Verification items for the finished model (mm, model axes). Face numbers are marked on the shaded views. A direction names the side the tool comes from. Coordinates: 2 decimals unless noted, no trailing zeros. Order: outer loops, then holes, each group sorted by start corner. A loop starts at its lowest first (then second) coordinate and runs counter-clockwise, first axis right, second up.
Q1. Thickness scan on line 1 (X direction, y = 13, z = 11.5); line 2 (X direction, y = 12, z = 27.5); line 3 (Z direction, x = 9, y = -3.5). Record the ranges inside material, lowest first.
Q2. Draft check along Y on the marked faces 1, 2, 3 and 4. Enter one of: pulls with the +Y half, pulls with the -Y half, needs draft (parallel to the pull), parting line crosses it, or undercut.
Q3. Cross-section at C-C, the plane y = -9. Record the boundary of the cut face in (x, z), and give its area (3 significant figures).
Q4. Cross-section at A-A, the plane z = 35. Record the boundary of the cut face in (x, y).
Q5. Depth check by flat-ended pin: P1, Ø2, axis at x = 12, z = 39, coming from the -Y side; P2, Ø2, axis at x = 6.5, z = 49, coming from the -Y side; P3, Ø2, axis at x = -5, y = -10.5, coming from the -Z side. Enter the tip coordinate at first touch or a pass-through.
Q6. Cross-section at D-D, the plane y = -13.5. Record the boundary of the cut face in (x, z), and give its area (3 significant figures).
Q7. Set-up check for the marked faces 5, 6, 7, 8 and 9: record each of +Z, -Z, +X, -X, +Y, -Y from which the full face is reachable in a straight line by a thin tool's end or side.
Q8. Cross-section at B-B, the plane x = -4. Record the boundary of the cut face in (y, z), and give its area (3 significant figures).
from build123d import *

# Parameters (mm, degrees)
F1_DEPTH = 60
F2_T     = -1
F4_DEPTH = 59
F6_DEPTH = 2


with BuildPart() as f1:
    # F0 (on Top) → F1 (new body)
    with BuildSketch(Plane.XY):
        Polygon((-7.2654252801, 15), (-14.5308505601, 20), (-12.0207078615, 11.5450849719), (-10.8981379201, 15), align=None)
        Polygon((-10.8981379201, 15), (-12.0207078615, 11.5450849719), (-9.510565163, 3.0901699437), (-16.5109876273, -2.2745751406), (-17.6335575688, -5.7294901688), (-14.6946313073, -7.8647450844), (-5.8778525229, -8.0901699437), (-2.9389262615, -16.4057647469), (0, -18.5410196625), (2.9389262615, -16.4057647469), (5.8778525229, -8.0901699437), (14.6946313073, -7.8647450844), (17.6335575688, -5.7294901688), (16.5109876273, -2.2745751406), (9.510565163, 3.0901699437), (12.0207078615, 11.5450849719), (10.8981379201, 15), (7.2654252801, 15), (0, 10), (-7.2654252801, 15), align=None)
        Polygon((-9.510565163, 3.0901699437), (-12.0207078615, 11.5450849719), (-16.5109876273, -2.2745751406), align=None)
        Polygon((7.2654252801, 15), (-7.2654252801, 15), (0, 10), align=None)
        Polygon((-17.6335575688, -5.7294901688), (-16.5109876273, -2.2745751406), (-23.5114100917, -7.639320225), (-14.6946313073, -7.8647450844), align=None)
        Polygon((14.5308505601, 20), (7.2654252801, 15), (10.8981379201, 15), (12.0207078615, 11.5450849719), align=None)
        Polygon((-5.8778525229, -8.0901699437), (-14.6946313073, -7.8647450844), (-2.9389262615, -16.4057647469), align=None)
        Polygon((16.5109876273, -2.2745751406), (12.0207078615, 11.5450849719), (9.510565163, 3.0901699437), align=None)
        Polygon((0, -18.5410196625), (-2.9389262615, -16.4057647469), (0, -24.72135955), (2.9389262615, -16.4057647469), align=None)
        Polygon((23.5114100917, -7.639320225), (16.5109876273, -2.2745751406), (17.6335575688, -5.7294901688), (14.6946313073, -7.8647450844), align=None)
        Polygon((5.8778525229, -8.0901699437), (2.9389262615, -16.4057647469), (14.6946313073, -7.8647450844), align=None)
    extrude(amount=F1_DEPTH)

    # F2
    f2_openings = [f1.faces().sort_by_distance(p)[0] for p in [
        (0, 0, 0),
    ]]
    offset(amount=F2_T, openings=f2_openings, kind=Kind.INTERSECTION)

    # F3 (on face) → F4 (join, through all)
    with BuildSketch(Plane(origin=(0, 0, 59), x_dir=(1, 0, 0), z_dir=(0, 0, -1))):
        Polygon((-15.6559881063, 2.8792251681), (-14.3583265336, 6.8730168274), (-20.6573081254, 6.7119662811), align=None)
        Polygon((0, 21.7203791484), (-2.0996605306, 15.7794590151), (2.0996605306, 15.7794590151), align=None)
        Polygon((20.6573081254, 6.7119662811), (14.3583265336, 6.8730168274), (15.6559881063, 2.8792251681), align=None)
        Polygon((12.7669185376, -17.5721558553), (10.9735943499, -11.5317010106), (7.5762722465, -14), align=None)
        Polygon((-7.5762722465, -14), (-10.9735943499, -11.5317010106), (-12.7669185376, -17.5721558553), align=None)
    extrude(amount=F4_DEPTH)

    # F5 (on face) → F6 (join)
    with BuildSketch(Plane(origin=(0, 0, 59), x_dir=(1, 0, 0), z_dir=(0, 0, -1))):
        with BuildLine():
            ThreePointArc((-1.9818535798, 1.8771366278), (-2.208391982, 1.6044906934), (-2.3976894584, 1.3047876426))
            Line((-2.3976894584, 1.3047876426), (-1.3090169944, 0.9510565163))
            Line((-1.3090169944, 0.9510565163), (-1.9818535798, 1.8771366278))
        make_face()
        with BuildLine():
            Line((-1.3090169944, 0.9510565163), (-2.3976894584, 1.3047876426))
            ThreePointArc((-2.3976894584, 1.3047876426), (-2.5961204766, 0.8435306766), (-2.7067064528, 0.3537311263))
            Line((-2.7067064528, 0.3537311263), (-1.6180339887, 0))
            Line((-1.6180339887, 0), (-2.7067064528, -0.3537311263))
            ThreePointArc((-2.7067064528, -0.3537311263), (-2.5961204766, -0.8435306766), (-2.3976894584, -1.3047876426))
            Line((-2.3976894584, -1.3047876426), (-1.3090169944, -0.9510565163))
            Line((-1.3090169944, -0.9510565163), (-1.9818535798, -1.8771366278))
            ThreePointArc((-1.9818535798, -1.8771366278), (-1.6044906934, -2.208391982), (-1.1728365854, -2.4649218801))
            Line((-1.1728365854, -2.4649218801), (-0.5, -1.5388417686))
            Line((-0.5, -1.5388417686), (-0.5, -2.6835397391))
            ThreePointArc((-0.5, -2.6835397391), (1.21e-08, -2.7297226107), (0.5000000237, -2.6835397347))
            Line((0.5000000237, -2.6835397347), (0.5000000237, -1.5388418013))
            Line((0.5000000237, -1.5388418013), (1.1728365854, -2.4649218801))
            ThreePointArc((1.1728365854, -2.4649218801), (1.6044906934, -2.208391982), (1.9818535798, -1.8771366278))
            Line((1.9818535798, -1.8771366278), (1.3090169944, -0.9510565163))
            Line((1.3090169944, -0.9510565163), (2.3976894584, -1.3047876426))
            ThreePointArc((2.3976894584, -1.3047876426), (2.5961204766, -0.8435306766), (2.7067064528, -0.3537311263))
            Line((2.7067064528, -0.3537311263), (1.6180339887, 0))
            Line((1.6180339887, 0), (2.7067064528, 0.3537311263))
            ThreePointArc((2.7067064528, 0.3537311263), (2.5961204766, 0.8435306766), (2.3976894584, 1.3047876426))
            Line((2.3976894584, 1.3047876426), (1.3090169944, 0.9510565163))
            Line((1.3090169944, 0.9510565163), (1.9818535798, 1.8771366278))
            ThreePointArc((1.9818535798, 1.8771366278), (1.6044906934, 2.208391982), (1.1728365854, 2.4649218801))
            Line((1.1728365854, 2.4649218801), (0.5, 1.5388417686))
            Line((0.5, 1.5388417686), (0.5, 2.6835397391))
            ThreePointArc((0.5, 2.6835397391), (0, 2.7297226107), (-0.5, 2.6835397391))
            Line((-0.5, 2.6835397391), (-0.5, 1.5388417686))
            Line((-0.5, 1.5388417686), (-1.1728365854, 2.4649218801))
            ThreePointArc((-1.1728365854, 2.4649218801), (-1.6044906934, 2.208391982), (-1.9818535798, 1.8771366278))
            Line((-1.9818535798, 1.8771366278), (-1.3090169944, 0.9510565163))
        make_face()
        with BuildLine():
            Line((-1.6180339887, 0), (-2.7067064528, 0.3537311263))
            ThreePointArc((-2.7067064528, 0.3537311263), (-2.7297226107, 0), (-2.7067064528, -0.3537311263))
            Line((-2.7067064528, -0.3537311263), (-1.6180339887, 0))
        make_face()
        with BuildLine():
            ThreePointArc((-0.5, 2.6835397391), (-0.8435306766, 2.5961204766), (-1.1728365854, 2.4649218801))
            Line((-1.1728365854, 2.4649218801), (-0.5, 1.5388417686))
            Line((-0.5, 1.5388417686), (-0.5, 2.6835397391))
        make_face()
        with BuildLine():
            Line((-1.3090169944, -0.9510565163), (-2.3976894584, -1.3047876426))
            ThreePointArc((-2.3976894584, -1.3047876426), (-2.208391982, -1.6044906934), (-1.9818535798, -1.8771366278))
            Line((-1.9818535798, -1.8771366278), (-1.3090169944, -0.9510565163))
        make_face()
        with BuildLine():
            ThreePointArc((1.1728365854, 2.4649218801), (0.8435306766, 2.5961204766), (0.5, 2.6835397391))
            Line((0.5, 2.6835397391), (0.5, 1.5388417686))
            Line((0.5, 1.5388417686), (1.1728365854, 2.4649218801))
        make_face()
        with BuildLine():
            Line((-0.5, -1.5388417686), (-1.1728365854, -2.4649218801))
            ThreePointArc((-1.1728365854, -2.4649218801), (-0.8435306766, -2.5961204766), (-0.5, -2.6835397391))
            Line((-0.5, -2.6835397391), (-0.5, -1.5388417686))
        make_face()
        with BuildLine():
            ThreePointArc((2.3976894584, 1.3047876426), (2.208391982, 1.6044906934), (1.9818535798, 1.8771366278))
            Line((1.9818535798, 1.8771366278), (1.3090169944, 0.9510565163))
            Line((1.3090169944, 0.9510565163), (2.3976894584, 1.3047876426))
        make_face()
        with BuildLine():
            Line((0.5000000237, -1.5388418013), (0.5000000237, -2.6835397347))
            ThreePointArc((0.5000000237, -2.6835397347), (0.8435306881, -2.5961204728), (1.1728365854, -2.4649218801))
            Line((1.1728365854, -2.4649218801), (0.5000000237, -1.5388418013))
        make_face()
        with BuildLine():
            ThreePointArc((2.7297226107, 0), (2.7239624938, 0.1772395647), (2.7067064528, 0.3537311263))
            Line((2.7067064528, 0.3537311263), (1.6180339887, 0))
            Line((1.6180339887, 0), (2.7067064528, -0.3537311263))
            ThreePointArc((2.7067064528, -0.3537311263), (2.7239624938, -0.1772395647), (2.7297226107, 0))
        make_face()
        with BuildLine():
            Line((1.3090169944, -0.9510565163), (1.9818535798, -1.8771366278))
            ThreePointArc((1.9818535798, -1.8771366278), (2.208391982, -1.6044906934), (2.3976894584, -1.3047876426))
            Line((2.3976894584, -1.3047876426), (1.3090169944, -0.9510565163))
        make_face()
        with BuildLine():
            Line((-2.3976894584, 1.3047876426), (-14.8526488228, 5.3516492559))
            Line((-14.8526488228, 5.3516492559), (-15.1616658171, 4.4005927396))
            Line((-15.1616658171, 4.4005927396), (-2.7067064528, 0.3537311263))
            ThreePointArc((-2.7067064528, 0.3537311263), (-2.5961204766, 0.8435306766), (-2.3976894584, 1.3047876426))
        make_face()
        with BuildLine():
            Line((-8.6335020293, 11.0323452951), (-1.9818535798, 1.8771366278))
            ThreePointArc((-1.9818535798, 1.8771366278), (-1.6044906934, 2.208391982), (-1.1728365854, 2.4649218801))
            Line((-1.1728365854, 2.4649218801), (-7.8244850349, 11.6201305474))
            Line((-7.8244850349, 11.6201305474), (-8.6335020293, 11.0323452951))
        make_face()
        with BuildLine():
            Line((-0.5, 15.7794590151), (-0.5, 2.6835397391))
            ThreePointArc((-0.5, 2.6835397391), (0, 2.7297226107), (0.5, 2.6835397391))
            Line((0.5, 2.6835397391), (0.5, 15.7794590151))
            Line((0.5, 15.7794590151), (-0.5, 15.7794590151))
        make_face()
        with BuildLine():
            Line((7.8244850349, 11.6201305474), (1.1728365854, 2.4649218801))
            ThreePointArc((1.1728365854, 2.4649218801), (1.6044906934, 2.208391982), (1.9818535798, 1.8771366278))
            Line((1.9818535798, 1.8771366278), (8.6335020293, 11.0323452951))
            Line((8.6335020293, 11.0323452951), (7.8244850349, 11.6201305474))
        make_face()
        with BuildLine():
            Line((14.8526488228, 5.3516492559), (2.3976894584, 1.3047876426))
            ThreePointArc((2.3976894584, 1.3047876426), (2.5961204766, 0.8435306766), (2.7067064528, 0.3537311263))
            Line((2.7067064528, 0.3537311263), (15.1616658171, 4.4005927396))
            Line((15.1616658171, 4.4005927396), (14.8526488228, 5.3516492559))
        make_face()
        with BuildLine():
            Line((13.4692997253, -3.8507096631), (2.7067064528, -0.3537311263))
            ThreePointArc((2.7067064528, -0.3537311263), (2.5961204766, -0.8435306766), (2.3976894584, -1.3047876426))
            Line((2.3976894584, -1.3047876426), (13.1602827309, -4.8017661794))
            Line((13.1602827309, -4.8017661794), (13.4692997253, -3.8507096631))
        make_face()
        with BuildLine():
            ThreePointArc((1.9818535798, -1.8771366278), (1.6044906934, -2.208391982), (1.1728365854, -2.4649218801))
            Line((1.1728365854, -2.4649218801), (8.8704248011, -13.0597431314))
            Line((8.8704248011, -13.0597431314), (9.6794417954, -12.4719578791))
            Line((9.6794417954, -12.4719578791), (1.9818535798, -1.8771366278))
        make_face()
        with BuildLine():
            ThreePointArc((0.5000000237, -2.6835397347), (1.21e-08, -2.7297226107), (-0.5, -2.6835397391))
            Line((-0.5, -2.6835397391), (-0.5, -14))
            Line((-0.5, -14), (0.5000000237, -14))
            Line((0.5000000237, -14), (0.5000000237, -2.6835397347))
        make_face()
        with BuildLine():
            ThreePointArc((-1.1728365854, -2.4649218801), (-1.6044906934, -2.208391982), (-1.9818535798, -1.8771366278))
            Line((-1.9818535798, -1.8771366278), (-9.6794417954, -12.4719578791))
            Line((-9.6794417954, -12.4719578791), (-8.8704248011, -13.0597431314))
            Line((-8.8704248011, -13.0597431314), (-1.1728365854, -2.4649218801))
        make_face()
        with BuildLine():
            ThreePointArc((-2.3976894584, -1.3047876426), (-2.5961204766, -0.8435306766), (-2.7067064528, -0.3537311263))
            Line((-2.7067064528, -0.3537311263), (-13.4692997253, -3.8507096631))
            Line((-13.4692997253, -3.8507096631), (-13.1602827309, -4.8017661794))
            Line((-13.1602827309, -4.8017661794), (-2.3976894584, -1.3047876426))
        make_face()
    extrude(amount=F6_DEPTH)


solid = f1.part
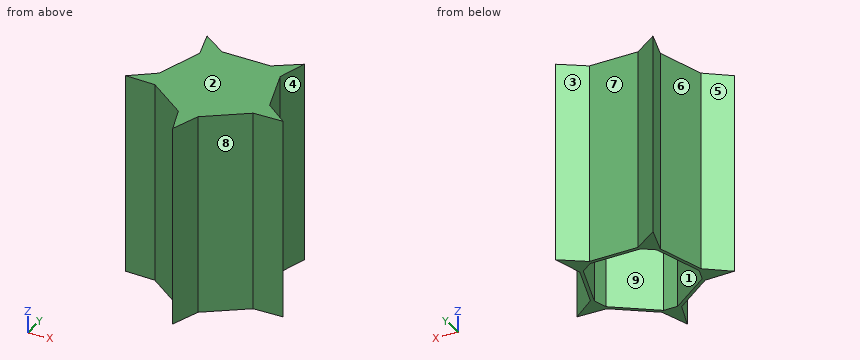
Check values:
1. line 1: x = -12.45 to -8.95, 8.95 to 12.45
1. line 2: x = -12.16 to -10.33, 10.33 to 12.16
1. line 3: z = 59 to 60
2. face 1: undercut
2. face 2: needs draft
2. face 3: pulls with the +Y half
2. face 4: undercut
3. outline: (-13.13, 0) - (-11.43, 0) - (-11.43, 59) - (-7.16, 59) - (-7.16, 57) - (-5.92, 57) - (-5.92, 59) - (-0.5, 59) - (-0.5, 57) - (0.5, 57) - (0.5, 59) - (5.92, 59) - (5.92, 57) - (7.16, 57) - (7.16, 59) - (11.43, 59) - (11.43, 0) - (13.13, 0) - (13.13, 60) - (-13.13, 60) - close
3. area: 234 mm2
4. outline: (-23.51, -7.64) - (-14.69, -7.86) - (-2.94, -16.41) - (0, -24.72) - (2.94, -16.41) - (14.69, -7.86) - (23.51, -7.64) - (16.51, -2.27) - (12.02, 11.55) - (14.53, 20) - (7.27, 15) - (-7.27, 15) - (-14.53, 20) - (-12.02, 11.55) - (-16.51, -2.27) - close; hole (-15.66, -2.88) - (-14.36, -6.87) - (-2.1, -15.78) - (2.1, -15.78) - (14.36, -6.87) - (15.66, -2.88) - (10.97, 11.53) - (7.58, 14) - (-7.58, 14) - (-10.97, 11.53) - close
5. P1: stops at y = -10.55
5. P2: stops at y = -14.55
5. P3: stops at z = 59
6. outline: (-6.94, 0) - (-5.24, 0) - (-5.24, 59) - (-0.5, 59) - (-0.5, 57) - (0.5, 57) - (0.5, 59) - (5.24, 59) - (5.24, 0) - (6.94, 0) - (6.94, 60) - (-6.94, 60) - close
6. area: 217 mm2
7. face 5: +Z, -Z, -X, +Y
7. face 6: +Z, -Z, -X
7. face 7: +Z, -Z, +Y
7. face 8: +Z, -Z, +X, -Y
7. face 9: -Z
8. outline: (-15.63, 0) - (-14.4, 0) - (-14.4, 59) - (-6.36, 59) - (-6.36, 57) - (-4.65, 57) - (-4.65, 59) - (-1.83, 59) - (-1.83, 57) - (-0.77, 57) - (-0.77, 59) - (0.77, 59) - (0.77, 57) - (1.83, 57) - (1.83, 59) - (4.65, 59) - (4.65, 57) - (6.36, 57) - (6.36, 59) - (14, 59) - (14, 0) - (15, 0) - (15, 60) - (-15.63, 60) - close
8. area: 174 mm2
